```python
from build123d import *

# Parameters (mm, degrees)
SKETCH_1_R               = 6
EXTRUDE_1_DEPTH          = 20
SKETCH_2_R               = 6.1
EXTRUDE_2_DEPTH          = 11
SKETCH_3_R               = 3.4
CUT_EXTRUDE_1_DEPTH      = 60.989832472
CUT_EXTRUDE_5_DEPTH      = 63.271823484
CUT_EXTRUDE_START        = -12
CUT_EXTRUDE_6_DEPTH      = 12
SKETCH_12_R              = 4
CUT_EXTRUDE_7_DEPTH      = 60.344586948
SKETCH_13_R              = 6.5
CUT_EXTRUDE_8_DEPTH      = 1
CUT_EXTRUDE_9_DEPTH      = 60.344586948
CUT_EXTRUDE_9_DEPTH_BACK = 60.344586948
CUT_EXTRUDE_10_DEPTH     = 2
CHAMFER_1_SIZE           = 0.2
M5X0_8_2_OUTLINE_R       = 2.1
M5X0_8_2_DEPTH           = 6
M5X0_8_2_2_OUTLINE_W     = 1.999932927
M5X0_8_2_2_OUTLINE_H     = 6.060126363


# Read off the part's stored shape, not the designer's step: M5x0.8 螺纹孔2
with BuildPart() as part:
    # 草图1 → 凸台-拉伸1 (new body)
    with BuildSketch(Plane(origin=(0, 0, 0), x_dir=(1, 0, 0), z_dir=(0, 1, 0))):
        with BuildLine():
            Line((0, 41.7), (0, 10.918333206))
            ThreePointArc((0, 10.918333206), (-0.463653568, 9.637849063), (-1.63963964, 8.951065962))
            ThreePointArc((-1.63963964, 8.951065962), (-9.1, 0), (-1.63963964, -8.951065962))
            ThreePointArc((-1.63963964, -8.951065962), (-0.463653568, -9.637849063), (0, -10.918333206))
            Line((0, -10.918333206), (0, -41.7))
            ThreePointArc((0, -41.7), (41.7, 0), (0, 41.7))
        make_face()
        with Locations(Location((0, 0, 0), (0, 0, 270))):
            Circle(SKETCH_1_R, mode=Mode.SUBTRACT)
    extrude(amount=EXTRUDE_1_DEPTH)

    # 草图2 → 凸台-拉伸2 (add)
    with BuildSketch(Plane.XZ):
        Circle(SKETCH_2_R)
    extrude(amount=-EXTRUDE_2_DEPTH)

    # 草图3 → 切除-拉伸1 (cut, through all)
    with BuildSketch(Plane(origin=(0, 11, 0), x_dir=(1, 0, 0), z_dir=(0, 1, 0))):
        with Locations(Location((0, 0, 0), (0, 0, 270))):
            Circle(SKETCH_3_R)
    extrude(amount=-CUT_EXTRUDE_1_DEPTH, mode=Mode.SUBTRACT)

    # 草图10 → 切除-拉伸5 (cut, through all)
    with BuildSketch(Plane.XZ):
        with BuildLine():
            Line((40.483206395, 10), (40.483206395, -10))
            ThreePointArc((40.483206395, -10), (41.394683878, -5.036878663), (41.7, 0))
            ThreePointArc((41.7, 0), (41.394683878, 5.036878663), (40.483206395, 10))
        make_face()
    extrude(amount=-CUT_EXTRUDE_5_DEPTH, mode=Mode.SUBTRACT)

    # 草图11 → 切除-拉伸6 (cut)
    with BuildSketch(Plane(origin=(0, 20, 0), x_dir=(1, 0, 0), z_dir=(0, 1, 0)).offset(CUT_EXTRUDE_START)):
        with BuildLine():
            Line((6, -36.124783736), (6, -6.841783393))
            ThreePointArc((6, -6.841783393), (9.1, 0), (6, 6.841783393))
            Line((6, 6.841783393), (6, 36.124783736))
            ThreePointArc((6, 36.124783736), (6.747974614, 37.684409471), (8.432432432, 38.077474749))
            ThreePointArc((8.432432432, 38.077474749), (39, 0), (8.432432432, -38.077474749))
            ThreePointArc((8.432432432, -38.077474749), (6.747974614, -37.684409471), (6, -36.124783736))
        make_face()
    extrude(amount=CUT_EXTRUDE_6_DEPTH, mode=Mode.SUBTRACT)

    # 草图12 → 切除-拉伸7 (cut, through all)
    with BuildSketch(Plane(origin=(0, 8, 0), x_dir=(1, 0, 0), z_dir=(0, 1, 0))):
        with Locations(Location((16, 0, 0), (0, 0, 270))):
            Circle(SKETCH_12_R)
    extrude(amount=-CUT_EXTRUDE_7_DEPTH, mode=Mode.SUBTRACT)

    # 草图13 → 切除-拉伸8 (cut)
    with BuildSketch(Plane(origin=(0, 8, 0), x_dir=(1, 0, 0), z_dir=(0, 1, 0))):
        with Locations(Location((16, 0, 0), (0, 0, 270))):
            Circle(SKETCH_13_R)
    extrude(amount=-CUT_EXTRUDE_8_DEPTH, mode=Mode.SUBTRACT)

    # 草图14 → 切除-拉伸9 (cut, two sides: drawn at the far end of the back side and taken through both)
    with BuildSketch(Plane(origin=(0, 8, 0), x_dir=(1, 0, 0), z_dir=(0, 1, 0)).offset(-CUT_EXTRUDE_9_DEPTH_BACK)):
        with BuildLine():
            ThreePointArc((22.891243611, 20.998113284), (30.339314214, 16.81648203), (35.645345475, 10.122766478))
            ThreePointArc((35.645345475, 10.122766478), (34.525042064, 6.62063566), (31.022911246, 7.740939071))
            ThreePointArc((31.022911246, 7.740939071), (26.965357928, 12.859662729), (21.269774526, 16.057380747))
            ThreePointArc((21.269774526, 16.057380747), (19.6101428, 19.338481558), (22.891243611, 20.998113284))
        make_face()
    extrude(amount=CUT_EXTRUDE_9_DEPTH + CUT_EXTRUDE_9_DEPTH_BACK, mode=Mode.SUBTRACT)

    # 草图15 → 切除-拉伸10 (cut)
    with BuildSketch(Plane(origin=(0, 8, 0), x_dir=(1, 0, 0), z_dir=(0, 1, 0))):
        with BuildLine():
            ThreePointArc((37.334311828, 10.993049569), (31.572105933, 18.262242929), (23.483703469, 22.803380942))
            ThreePointArc((23.483703469, 22.803380942), (17.804875142, 19.930941416), (20.677314668, 14.252113089))
            ThreePointArc((20.677314668, 14.252113089), (25.732566208, 11.413901831), (29.333944893, 6.87065598))
            ThreePointArc((29.333944893, 6.87065598), (35.395325154, 4.931669307), (37.334311828, 10.993049569))
        make_face()
    extrude(amount=-CUT_EXTRUDE_10_DEPTH, mode=Mode.SUBTRACT)

    # 倒角1
    chamfer_1_edges = [part.edges().sort_by_distance(p)[0] for p in [
        (0, 10, 41.7),
        (0, 10, -41.7),
    ]]
    chamfer(chamfer_1_edges, length=CHAMFER_1_SIZE)

    # M5x0.8 螺纹孔2 outline → M5x0.8 螺纹孔2 (cut)
    with BuildSketch(Plane.YZ):
        with Locations((15, -33.667083302)):
            Circle(M5X0_8_2_OUTLINE_R)
        with Locations((10, 20.918333206)):
            Circle(M5X0_8_2_OUTLINE_R)
        with Locations((15, 33.667083302)):
            Circle(M5X0_8_2_OUTLINE_R)
    extrude(amount=M5X0_8_2_DEPTH, mode=Mode.SUBTRACT)

    # M5x0.8 _2 2 outline → M5x0.8 _2 2 (revolve, cut)
    with BuildSketch(Plane(origin=(0, 10, -20.918333206), x_dir=(0, 1, 0), z_dir=(0, 0, -1))):
        with Locations((0.999966464, 3.030063182)):
            Rectangle(M5X0_8_2_2_OUTLINE_W, M5X0_8_2_2_OUTLINE_H)
        Polygon((2.100006439, 5.999996131), (1.999932927, 6.060126363), (1.999932927, 0), (2.100006439, 0), align=None)
    revolve(axis=Axis((0, 10, -20.918333206), (1, 0, 0)), mode=Mode.SUBTRACT)


solid = part.part
```
Geometry: final body of the model. Coordinates: model frame, mm. A direction names the side the tool comes from. Round coordinates to 2 decimals unless told otherwise and drop trailing zeros. Order: outer loops, then holes, each group sorted by start corner. A loop starts at its lowest first (then second) coordinate and runs counter-clockwise, first axis right, second up. Notation, with made-up numbers: (42.5, 3) - (79.5, 3) arc R23 cw to (79.5, 32) - close; hole circle Ø2 at (-35.75, -29). An arc over 180 degrees is marked (long way). Use CSV: the item, a comma, the result in double quotes. Start each with the question number.
Q1. Material intervals for line 1 along X through (y, z) = (8.75, 0); line 2 along X through (y, z) = (3.25, 0); line 3 along Z through (x, y) = (1.35, 10), sorted ascending. Write a range as from..to.
Q2. Section query C-C (y = 3.5). Return loops of the section in (x, z).
Q3. Section query A-A (y = 10). State how many separate pieces and enclosed holes the cut face has, and give its area (3 significant figures).
Q4. Access query for faces 1 (the face through (0, 10, -26)), 2 (the face through (6.73, 13.92, -37.67)), 3 (the face through (2.958, 14.727, -31.585)). Directions: +Z, -Z, +X, -X, +Y, -Y. A direction counts if a zero-diameter tool reaches every point of the face in a straight line with its end or side. Return the directions, or none.
Q5. Section query D-D (z = 34.5). Return loops of the section in (x, y), and give its area (3 significant figures).
Q6. Section query B-B (z = 0). Return loops of the section in (x, y), and give its area (3 significant figures).
Q7. Mould query, pull axis X, two halves, no side actions, for faces 4 (the face through (25.67, 7.014, -11.467)), 5 (the face through (0, 10, 26)), 6 (the face through (2.958, 8.334, 19.641)). Classes: +X half, -X half, draft (parallel to the pull), parting line (faces both ways), or undercut.
Q8. First-contact query: pin 1 (6.5 mm diameter, centred on x = 16, z = 0, fed in from +Y); pin 2 (4 mm diameter, centred on y = 16.5, z = 26.5, fed in from +X); pin 3 (4 mm diameter, centred on y = 13.5, z = -16.5, fed in from +X); pin 4 (1.5 mm diameter, centred on x = 26, y = 8.5, fed in from -Z). Flat tips, straight axial feed; report the tip coordinate or a pass-through.
Result set:
1,line 1,"x = -9.1..-3.4, 3.4..9.1, 39..40.48"
1,line 2,"x = -9.1..-3.4, 3.4..12, 20..40.48"
1,line 3,"z = -41.68..-23.02, -18.82..-3.12, 3.12..18.82, 23.02..41.68"
2,outline,"(-1.64, -8.95) arc R2 cw to (0, -10.92) - (0, -41.5) - (0.2, -41.7) arc R41.7 ccw to (40.48, -10) - (40.48, 10) arc R41.7 ccw to (0.2, 41.7) - (0, 41.5) - (0, 10.92) arc R2 cw to (-1.64, 8.95) arc R9.1 ccw to start; hole circle Ø6.8 at (0, 0); hole circle Ø8 at (16, 0); hole (21.27, -16.06) arc R2.6 ccw to (22.89, -21) arc R22.1 ccw to (35.65, -10.12) arc R2.6 ccw to (31.02, -7.74) arc R16.9 cw to start"
3,separate pieces,"2"
3,enclosed holes,"1"
3,area,"869 mm2"
4,face 1,"-Z, -X, +Y, -Y"
4,face 2,"+Y"
4,face 3,"-X"
5,outline,"(0, 0) - (23.42, 0) - (23.42, 20) - (18.19, 20) - (18.19, 8) - (6, 8) - (6, 13.07) - (0, 13.07) - close; (0, 16.93) - (6, 16.93) - (6, 20) - (0, 20) - close"
5,area,"299 mm2"
6,outline,"(-9.1, 0) - (-3.4, 0) - (-3.4, 11) - (-6, 11) - (-6, 20) - (-9.1, 20) - close; (3.4, 0) - (12, 0) - (12, 7) - (9.5, 7) - (9.5, 8) - (9.1, 8) - (9.1, 20) - (6, 20) - (6, 11) - (3.4, 11) - close; (20, 0) - (40.48, 0) - (40.48, 20) - (39, 20) - (39, 8) - (22.5, 8) - (22.5, 7) - (20, 7) - close"
6,area,"381 mm2"
7,face 4,"undercut"
7,face 5,"-X half"
7,face 6,"draft"
8,pin 1,"passes through"
8,pin 2,"stops at x = 33.74"
8,pin 3,"stops at x = 39.1"
8,pin 4,"stops at z = -33.19"
